CAD build for the part. Positions are in the model's coordinates, mm. A direction names the side the tool comes from. Round coordinates to 2 decimals unless told otherwise and drop trailing zeros. Loops run counter-clockwise (first coordinate to the right, second up) from the corner with the lowest first, then second, coordinate; pieces in that order, holes last.
```python
from build123d import *

# Parameters (mm, degrees)
BOSS_EXTRUDE1_DEPTH      = 35
CUT_EXTRUDE1_REACH       = 164.604
SKETCH2_W                = 42
SKETCH2_H                = 21
SKETCH3_R                = 2
CUT_EXTRUDE2_DEPTH       = 10
FILLET1_R                = 20
CUT_EXTRUDE5_REACH       = 164.604
SKETCH6_W                = 42
SKETCH6_H                = 9
CUT_EXTRUDE7_DEPTH       = 9
SKETCH9_R                = 2
CUT_EXTRUDE8_DEPTH       = 10
CUT_EXTRUDE9_DEPTH       = 6
SKETCH11_R               = 2
CUT_EXTRUDE10_DEPTH      = 9
SKETCH12_R               = 2
CUT_EXTRUDE11_DEPTH      = 10
SKETCH14_W               = 85
SKETCH14_H               = 33
CUT_EXTRUDE13_DEPTH      = 4
SKETCH15_W               = 28
SKETCH15_H               = 20
CUT_EXTRUDE14_DEPTH      = 4
BOSS_EXTRUDE2_DEPTH      = 5
BOSS_EXTRUDE2_DEPTH_BACK = 9
SKETCH16_W               = 80
SKETCH16_H               = 11
SKETCH13_R               = 2
CUT_EXTRUDE12_DEPTH      = 12
FILLET2_R                = 2
SKETCH17_W               = 28.5
SKETCH17_H               = 40
SKETCH17_W_2             = 18
SKETCH17_H_2             = 10
CUT_EXTRUDE15_DEPTH      = 8
CUT_EXTRUDE18_REACH      = 104.86
SKETCH20_W               = 8
SKETCH20_H               = 16
SKETCH7_R                = 2
CUT_EXTRUDE6_DEPTH       = 13
CHAMFER1_SIZE            = 10
CHAMFER1_SIZE2           = 3.639702343
CUT_EXTRUDE19_REACH      = 164.604
SKETCH22_W               = 7
SKETCH22_H               = 14
BOSS_EXTRUDE4_REACH      = 141.461
BOSS_EXTRUDE5_START      = -3
BOSS_EXTRUDE5_DEPTH      = 3
CUT_EXTRUDE21_DEPTH      = 140.460664257
SKETCH27_W               = 7.175165893
SKETCH27_H               = 9
CUT_EXTRUDE22_DEPTH      = 140.460664257
SKETCH28_W               = 5
SKETCH28_H               = 2
BOSS_EXTRUDE6_DEPTH      = 2
SKETCH29_W               = 4
SKETCH29_H               = 8
BOSS_EXTRUDE7_DEPTH      = 1
SKETCH30_W               = 3
SKETCH30_H               = 7
BOSS_EXTRUDE8_DEPTH      = 2


with BuildPart() as part:
    # Sketch1 → Boss-Extrude1 (new body)
    with BuildSketch(Plane(origin=(0, 0, 0), x_dir=(1, 0, 0), z_dir=(0, 1, 0))):
        Polygon((-40.317617866, 43.23325062), (45.682382134, 43.23325062), (45.682382134, -16.76674938), (65.682382134, -16.76674938), (65.682382134, 118.23325062), (45.682382134, 118.23325062), (45.682382134, 58.23325062), (-40.317617866, 58.23325062), align=None)
    extrude(amount=BOSS_EXTRUDE1_DEPTH)

    # Sketch2 → Cut-Extrude1 (cut, up to next)
    with BuildSketch(Plane(origin=(65.682382134, 0, 0), x_dir=(0, 0, -1), z_dir=(1, 0, 0)), mode=Mode.PRIVATE) as cut_extrude1_sk1:
        with Locations((13.23325062, 19.5)):
            Rectangle(SKETCH2_W, SKETCH2_H)
    cut_extrude1_tool1 = extrude(cut_extrude1_sk1.sketch, amount=-CUT_EXTRUDE1_REACH, mode=Mode.PRIVATE) & part.part
    # Sketch2 → Cut-Extrude1 (cut, up to next)
    with BuildSketch(Plane(origin=(65.682382134, 0, 0), x_dir=(0, 0, -1), z_dir=(1, 0, 0)), mode=Mode.PRIVATE) as cut_extrude1_sk2:
        with Locations((88.23325062, 19.5)):
            Rectangle(SKETCH2_W, SKETCH2_H)
    cut_extrude1_tool2 = extrude(cut_extrude1_sk2.sketch, amount=-CUT_EXTRUDE1_REACH, mode=Mode.PRIVATE) & part.part
    add(cut_extrude1_tool1.solids().sort_by_distance((65.682382, 19.5, -13.233251))[0], mode=Mode.SUBTRACT)
    add(cut_extrude1_tool2.solids().sort_by_distance((65.682382, 19.5, -88.233251))[0], mode=Mode.SUBTRACT)

    # Sketch3 → Cut-Extrude2 (cut)
    with BuildSketch(Plane.ZY.offset(-45.682382134)):
        with Locations((11.26674938, 24.75)):
            Circle(SKETCH3_R)
        with Locations((11.26674938, 15.25)):
            Circle(SKETCH3_R)
        with Locations((-37.73325062, 24.75)):
            Circle(SKETCH3_R)
        with Locations((-37.73325062, 15.25)):
            Circle(SKETCH3_R)
        with Locations(Location((-112.73325062, 24.75, 0), (0, 0, 180))):
            Circle(SKETCH3_R)
        with Locations(Location((-112.73325062, 15.25, 0), (0, 0, 180))):
            Circle(SKETCH3_R)
        with Locations(Location((-63.73325062, 15.25, 0), (0, 0, 180))):
            Circle(SKETCH3_R)
        with Locations(Location((-63.73325062, 24.75, 0), (0, 0, 180))):
            Circle(SKETCH3_R)
    extrude(amount=-CUT_EXTRUDE2_DEPTH, mode=Mode.SUBTRACT)

    # Fillet1
    fillet1_edges = [part.edges().sort_by_distance(p)[0] for p in [
        (55.682382134, 0, -118.23325062),
        (55.682382134, 0, 16.76674938),
    ]]
    fillet(fillet1_edges, radius=FILLET1_R)

    # Sketch6 → Cut-Extrude5 (cut, up to next)
    with BuildSketch(Plane(origin=(65.682382134, 0, 0), x_dir=(0, 0, -1), z_dir=(1, 0, 0)), mode=Mode.PRIVATE) as cut_extrude5_sk1:
        with Locations((13.23325062, 4.5)):
            Rectangle(SKETCH6_W, SKETCH6_H)
    cut_extrude5_tool1 = extrude(cut_extrude5_sk1.sketch, amount=-CUT_EXTRUDE5_REACH, mode=Mode.PRIVATE) & part.part
    # Sketch6 → Cut-Extrude5 (cut, up to next)
    with BuildSketch(Plane(origin=(65.682382134, 0, 0), x_dir=(0, 0, -1), z_dir=(1, 0, 0)), mode=Mode.PRIVATE) as cut_extrude5_sk2:
        with Locations((88.23325062, 4.5)):
            Rectangle(SKETCH6_W, SKETCH6_H)
    cut_extrude5_tool2 = extrude(cut_extrude5_sk2.sketch, amount=-CUT_EXTRUDE5_REACH, mode=Mode.PRIVATE) & part.part
    add(cut_extrude5_tool1.solids().sort_by_distance((65.682382, 4.5, -13.233251))[0], mode=Mode.SUBTRACT)
    add(cut_extrude5_tool2.solids().sort_by_distance((65.682382, 4.5, -88.233251))[0], mode=Mode.SUBTRACT)

    # Sketch8 → Cut-Extrude7 (cut)
    with BuildSketch(Plane.XZ):
        Polygon((45.682382134, -67.23325062), (45.682382134, -58.23325062), (25.682382134, -58.23325062), (25.682382134, -43.23325062), (45.682382134, -43.23325062), (45.682382134, -34.23325062), (65.682382134, -34.23325062), (65.682382134, -67.23325062), align=None)
    extrude(amount=-CUT_EXTRUDE7_DEPTH, mode=Mode.SUBTRACT)

    # Sketch9 → Cut-Extrude8 (cut)
    with BuildSketch(Plane.XZ.offset(-9)):
        with Locations(Location((55.682382134, -42.23325062, 0), (0, 0, 270))):
            Circle(SKETCH9_R)
        with Locations(Location((55.682382134, -59.23325062, 0), (0, 0, 270))):
            Circle(SKETCH9_R)
    extrude(amount=-CUT_EXTRUDE8_DEPTH, mode=Mode.SUBTRACT)

    # Sketch10 → Cut-Extrude9 (cut)
    with BuildSketch(Plane(origin=(0, 35, 0), x_dir=(1, 0, 0), z_dir=(0, 1, 0))):
        Polygon((45.682382134, 62.23325062), (65.682382134, 62.23325062), (65.682382134, 39.23325062), (45.682382134, 39.23325062), (45.682382134, 43.23325062), (43.682382134, 43.23325062), (43.682382134, 58.23325062), (45.682382134, 58.23325062), align=None)
    extrude(amount=-CUT_EXTRUDE9_DEPTH, mode=Mode.SUBTRACT)

    # Sketch11 → Cut-Extrude10 (cut)
    with BuildSketch(Plane(origin=(0, 29, 0), x_dir=(1, 0, 0), z_dir=(0, 1, 0))):
        with Locations(Location((55.682382134, 58.23325062, 0), (0, 0, 270))):
            Circle(SKETCH11_R)
        with Locations(Location((55.682382134, 43.23325062, 0), (0, 0, 270))):
            Circle(SKETCH11_R)
    extrude(amount=-CUT_EXTRUDE10_DEPTH, mode=Mode.SUBTRACT)

    # Sketch12 → Cut-Extrude11 (cut)
    with BuildSketch(Plane(origin=(0, 35, 0), x_dir=(1, 0, 0), z_dir=(0, 1, 0))):
        with Locations(Location((60.682382134, -11.76674938, 0), (0, 0, 270))):
            Circle(SKETCH12_R)
        with Locations(Location((60.682382134, 113.23325062, 0), (0, 0, 270))):
            Circle(SKETCH12_R)
    extrude(amount=-CUT_EXTRUDE11_DEPTH, mode=Mode.SUBTRACT)

    # Sketch14 → Cut-Extrude13 (cut)
    with BuildSketch(Plane.XY.offset(-43.23325062)):
        with Locations((2.182382134, 16.5)):
            Rectangle(SKETCH14_W, SKETCH14_H)
    extrude(amount=-CUT_EXTRUDE13_DEPTH, mode=Mode.SUBTRACT)

    # Sketch15 → Cut-Extrude14 (cut)
    with BuildSketch(Plane.XY.offset(-47.23325062)):
        with Locations((29.682382134, 10)):
            Rectangle(SKETCH15_W, SKETCH15_H)
    extrude(amount=-CUT_EXTRUDE14_DEPTH, mode=Mode.SUBTRACT)

    # Sketch16 → Boss-Extrude2 (add, two sides: drawn at the far end of the back side and taken through both)
    with BuildSketch(Plane.XZ.offset(-BOSS_EXTRUDE2_DEPTH_BACK)):
        with Locations((-0.317617866, -52.73325062)):
            Rectangle(SKETCH16_W, SKETCH16_H)
    extrude(amount=BOSS_EXTRUDE2_DEPTH + BOSS_EXTRUDE2_DEPTH_BACK)

    # Sketch13 → Cut-Extrude12 (cut)
    with BuildSketch(Plane.XY.offset(-43.23325062)):
        with Locations((-28.317617866, 29.5)):
            Circle(SKETCH13_R)
        with Locations((34.182382134, 29.5)):
            Circle(SKETCH13_R)
        with Locations((34.182382134, -1.5)):
            Circle(SKETCH13_R)
        with Locations((-28.317617866, -1.5)):
            Circle(SKETCH13_R)
    extrude(amount=-CUT_EXTRUDE12_DEPTH, mode=Mode.SUBTRACT)

    # Fillet2
    fillet2_edges = [part.edges().sort_by_distance(p)[0] for p in [
        (39.682382134, -5, -52.73325062),
    ]]
    fillet(fillet2_edges, radius=FILLET2_R)

    # Sketch17 → Cut-Extrude15 (cut)
    with BuildSketch(Plane.XY.offset(-43.23325062)):
        with Locations((29.432382134, 15)):
            Rectangle(SKETCH17_W, SKETCH17_H)
        with Locations((-0.317617866, 30)):
            Rectangle(SKETCH17_W_2, SKETCH17_H_2)
    extrude(amount=-CUT_EXTRUDE15_DEPTH, mode=Mode.SUBTRACT)

    # Sketch20 → Cut-Extrude18 (cut, up to next)
    with BuildSketch(Plane.XY.offset(-47.23325062), mode=Mode.PRIVATE) as cut_extrude18_sk1:
        with Locations((-36.317617866, 16.5)):
            Rectangle(SKETCH20_W, SKETCH20_H)
    cut_extrude18_tool1 = extrude(cut_extrude18_sk1.sketch, amount=-CUT_EXTRUDE18_REACH, mode=Mode.PRIVATE) & part.part
    add(cut_extrude18_tool1.solids().sort_by_distance((-36.317618, 16.5, -47.233251))[0], mode=Mode.SUBTRACT)

    # Sketch7 → Cut-Extrude6 (cut)
    with BuildSketch(Plane.ZY.offset(40.317617866)):
        with Locations((-50.73325062, 28.5)):
            Circle(SKETCH7_R)
        with Locations((-50.73325062, 5)):
            Circle(SKETCH7_R)
    extrude(amount=-CUT_EXTRUDE6_DEPTH, mode=Mode.SUBTRACT)

    # Chamfer1
    chamfer1_edges = [part.edges().sort_by_distance(p)[0] for p in [
        (-32.317617866, 16.5, -47.23325062),
    ]]
    chamfer1_side = [part.faces().sort_by_distance(p)[0] for p in [
        (-32.317617866, 16.5, -52.73325062),
    ]]
    chamfer(chamfer1_edges, length=CHAMFER1_SIZE, length2=CHAMFER1_SIZE2, reference=chamfer1_side[0])

    # Sketch22 → Cut-Extrude19 (cut, up to next)
    with BuildSketch(Plane(origin=(65.682382134, 0, 0), x_dir=(0, 0, -1), z_dir=(1, 0, 0)), mode=Mode.PRIVATE) as cut_extrude19_sk1:
        with Locations((46.73325062, 19)):
            Rectangle(SKETCH22_W, SKETCH22_H)
    cut_extrude19_tool1 = extrude(cut_extrude19_sk1.sketch, amount=-CUT_EXTRUDE19_REACH, mode=Mode.PRIVATE) & part.part
    add(cut_extrude19_tool1.solids().sort_by_distance((65.682382, 19, -46.733251))[0], mode=Mode.SUBTRACT)

    # Boss-Extrude4: up to this face of the body (flat: up to its plane)
    boss_extrude4_end = Plane(part.part.faces().sort_by_distance((54.930904304, 26, -46.8909066))[0])
    # Sketch24 → Boss-Extrude4 (add, up to the picked face)
    with BuildSketch(Plane(origin=(0, 29, 0), x_dir=(1, 0, 0), z_dir=(0, 1, 0)), mode=Mode.PRIVATE) as boss_extrude4_sk1:
        with BuildLine():
            Line((37.182382134, 51.23325062), (45.682382134, 51.23325062))
            Line((45.682382134, 51.23325062), (45.682382134, 39.23325062))
            ThreePointArc((45.682382134, 39.23325062), (43.342105313, 46.585971205), (37.182382134, 51.23325062))
        make_face()
    boss_extrude4_tool1 = split(extrude(boss_extrude4_sk1.sketch, amount=-BOSS_EXTRUDE4_REACH, mode=Mode.PRIVATE), bisect_by=boss_extrude4_end, keep=Keep.BOTH, mode=Mode.PRIVATE)
    add(boss_extrude4_tool1.solids().sort_by(Axis((43.397163, 29, -48.466484), (0, -1, 0)))[0])

    # Sketch25 → Boss-Extrude5 (add)
    with BuildSketch(Plane.XZ.offset(-9).offset(BOSS_EXTRUDE5_START)):
        with BuildLine():
            Line((37.182382134, -51.23325062), (45.682382134, -51.23325062))
            Line((45.682382134, -51.23325062), (45.682382134, -39.23325062))
            ThreePointArc((45.682382134, -39.23325062), (43.342105313, -46.585971205), (37.182382134, -51.23325062))
        make_face()
    extrude(amount=BOSS_EXTRUDE5_DEPTH)

    # Sketch26 → Cut-Extrude21 (cut, through all)
    with BuildSketch(Plane(origin=(0, 29, 0), x_dir=(1, 0, 0), z_dir=(0, 1, 0))):
        with BuildLine():
            Line((45.239754001, 42.559669232), (43.686053775, 42.559669232))
            Line((43.686053775, 42.559669232), (44.063234426, 45.443837008))
            ThreePointArc((44.063234426, 45.443837008), (44.740108693, 44.037901041), (45.239754001, 42.559669232))
        make_face()
    extrude(amount=-CUT_EXTRUDE21_DEPTH, mode=Mode.SUBTRACT)

    # Sketch27 → Cut-Extrude22 (cut, through all)
    with BuildSketch(Plane(origin=(0, 29, 0), x_dir=(1, 0, 0), z_dir=(0, 1, 0))):
        with Locations((42.937910719, 45.73325062)):
            Rectangle(SKETCH27_W, SKETCH27_H)
    extrude(amount=-CUT_EXTRUDE22_DEPTH, mode=Mode.SUBTRACT)

    # Sketch28 → Boss-Extrude6 (add)
    with BuildSketch(Plane.XY.offset(-47.23325062)):
        with Locations((-36.817617866, 30.5)):
            Rectangle(SKETCH28_W, SKETCH28_H)
        with Locations((-36.817617866, -2.5)):
            Rectangle(SKETCH28_W, SKETCH28_H)
    extrude(amount=BOSS_EXTRUDE6_DEPTH)

    # Sketch29 → Boss-Extrude7 (add)
    with BuildSketch(Plane.XY.offset(-51.23325062)):
        with Locations((36.182382134, 20.5)):
            Rectangle(SKETCH29_W, SKETCH29_H)
    extrude(amount=BOSS_EXTRUDE7_DEPTH)

    # Sketch30 → Boss-Extrude8 (add)
    with BuildSketch(Plane.XY.offset(-51.23325062)):
        with Locations((35.182382134, 8)):
            Rectangle(SKETCH30_W, SKETCH30_H)
    extrude(amount=BOSS_EXTRUDE8_DEPTH)


solid = part.part
```
Item 1: Probe line 1 (Z direction, x = 6, y = 27.5); line 2 (Z direction, x = 37.5, y = 17); line 3 (X direction, y = 15.5, z = -51.5). List the from-to ranges inside material, lowest first.
Answers follow:
line 1: z = -58.23 to -51.23
line 2: z = -58.23 to -50.23
line 3: x = -30.23 to 65.68
Item 2: Flat gauge pins, fed straight in: P1, Ø0.8, axis at x = 36, z = -50.5, coming from the -Y side; P2, Ø0.6, axis at x = -31.5, y = 34, coming from the +Z side; P3, Ø2, axis at y = 30, z = -46, coming from the -X side. Where does each tip first touch, or does it go through?
Answers follow:
P1: stops at y = 4.5
P2: stops at z = -43.23
P3: stops at x = -39.32
Item 3: Cut at A-A, the plane x = 1. Give the cut face in (y, z), plus the area to 3 significant figures.
Answers follow:
outline: (-5, -58.23) - (35, -58.23) - (35, -51.23) - (25, -51.23) - (25, -47.23) - (-5, -47.23) - close
area: 400 mm2
Item 4: Two-plate mould, pull along Y, no slides. Class faces 1 (the cylindrical face through (-33.91, 5.09, -52.73)), 2 (the flat face through (2, 15, -58.233)), 3 (the cylindrical face through (55.822, 10.392, 14.308)): released by +Y, released by -Y, zero draft, split by the parting line, or undercut.
Answers follow:
face 1: undercut
face 2: zero draft
face 3: released by -Y
Item 5: Cut at B-B, the plane z = -9. Give the cut face in (x, y), plus the area to 4 significant figures.
Answers follow:
outline: (45.68, 30) - (65.68, 30) - (65.68, 35) - (45.68, 35) - close
area: 100.0 mm2
Item 6: 3-axis set-ups, long thin cutter, end or side, ignore diameter. For faces 4 (the flat face through (-28, -1, -55.233)), 5 (the flat face through (55.682, 15, 11)), 6 (the flat face through (0, 30, -51.233)), 7 (the flat face through (56, 26, -47)), 8 (the flat face through (56, 16, -109.233)): which of +Z, -Z, +X, -X, +Y, -Y reach the whole face in a straight line?
Answers follow:
face 4: +Z
face 5: -X
face 6: +Z, +Y
face 7: +X
face 8: +X, -X, -Y
Item 7: Cut at C-C, the plane x = 23.5. Give the cut face in (y, z), plus the area to 3 significant figures.
Answers follow:
outline: (-5, -58.23) - (35, -58.23) - (35, -51.23) - (-5, -51.23) - close
area: 280 mm2
